Verification items for the finished model (mm, model axes). A direction names the side the tool comes from. Round coordinates to 2 decimals unless told otherwise and drop trailing zeros. Order: outer loops, then holes, each group sorted by start corner. A loop starts at its lowest first (then second) coordinate and runs counter-clockwise, first axis right, second up. Notation, with made-up numbers: M 74.5,73 L 105.5,73 A34 cw 105.5,105 Z; hole C 25,44 d7. An arc over 180 degrees is marked long. Write item = value, one per line. Start each with the question number.
from build123d import *

# Parameters (mm, degrees)
SKIZZE4_R                        = 5
SCHNITT_LINEAR_AUSTRAGEN1_DEPTH  = 32.25
SKIZZE5_R                        = 1.3
SCHNITT_LINEAR_AUSTRAGEN2_DEPTH  = 13
F_2_6_2_6_DURCHMESSER_BOHRUNG1_D = 2.6
KREISMUSTER1_COUNT               = 21


with BuildPart() as part:
    # Skizze2 → Rotation1 (revolve)
    with BuildSketch(Plane.XY, mode=Mode.PRIVATE) as rotation1_sk:
        Polygon((0, 26.075), (3.5, 26.075), (3.5, 41), (35.75, 41), (35.75, 50), (0, 50), align=None)
    rotation1 = revolve(rotation1_sk.sketch.rotate(Axis((0, 0, 0), (-1, 0, 0)), 90), axis=Axis((0, 0, 0), (-1, 0, 0)))

    # Skizze4 → Schnitt-Linear austragen1 (cut)
    with BuildSketch(Plane(origin=(35.75, 0, 0), x_dir=(0, 0, -1), z_dir=(1, 0, 0))):
        with Locations((40, 0)):
            Circle(SKIZZE4_R)
        with Locations((38.222912231, -11.790206976)):
            Circle(SKIZZE4_R)
        with Locations((33.049550973, -22.532802323)):
            Circle(SKIZZE4_R)
        with Locations((24.939592074, -31.273259299)):
            Circle(SKIZZE4_R)
        with Locations((14.613640975, -37.234949946)):
            Circle(SKIZZE4_R)
        with Locations((2.989203743, -39.888151887)):
            Circle(SKIZZE4_R)
        with Locations((-8.900837358, -38.997116487)):
            Circle(SKIZZE4_R)
        with Locations((-20, -34.641016151)):
            Circle(SKIZZE4_R)
        with Locations((-29.322074873, -27.206909511)):
            Circle(SKIZZE4_R)
        with Locations((-36.038754716, -17.355349565)):
            Circle(SKIZZE4_R)
        with Locations((-39.553233049, -5.961690647)):
            Circle(SKIZZE4_R)
        with Locations((-39.553233049, 5.961690647)):
            Circle(SKIZZE4_R)
        with Locations((-36.038754716, 17.355349565)):
            Circle(SKIZZE4_R)
        with Locations((-29.322074873, 27.206909511)):
            Circle(SKIZZE4_R)
        with Locations((-20, 34.641016151)):
            Circle(SKIZZE4_R)
        with Locations((-8.900837358, 38.997116487)):
            Circle(SKIZZE4_R)
        with Locations((2.989203743, 39.888151887)):
            Circle(SKIZZE4_R)
        with Locations((14.613640975, 37.234949946)):
            Circle(SKIZZE4_R)
        with Locations((24.939592074, 31.273259299)):
            Circle(SKIZZE4_R)
        with Locations((33.049550973, 22.532802323)):
            Circle(SKIZZE4_R)
        with Locations((38.222912231, 11.790206976)):
            Circle(SKIZZE4_R)
    schnitt_linear_austragen1 = extrude(amount=-SCHNITT_LINEAR_AUSTRAGEN1_DEPTH, mode=Mode.SUBTRACT)

    # Skizze5 → Schnitt-Linear austragen2 (cut)
    with BuildSketch(Plane(origin=(35.75, 0, 0), x_dir=(0, 0, -1), z_dir=(1, 0, 0))):
        with Locations((-46.369838758, 0)):
            Circle(SKIZZE5_R)
        with Locations((-28.91112158, 36.253399778)):
            Circle(SKIZZE5_R)
        with Locations((10.318259828, 45.207250089)):
            Circle(SKIZZE5_R)
        with Locations((41.777781131, 20.119119023)):
            Circle(SKIZZE5_R)
        with Locations((41.777781131, -20.119119023)):
            Circle(SKIZZE5_R)
        with Locations((10.318259828, -45.207250089)):
            Circle(SKIZZE5_R)
        with Locations((-28.91112158, -36.253399778)):
            Circle(SKIZZE5_R)
    schnitt_linear_austragen2 = extrude(amount=-SCHNITT_LINEAR_AUSTRAGEN2_DEPTH, mode=Mode.SUBTRACT)

    # Spiegeln1: Rotation1, Schnitt-Linear austragen1, Schnitt-Linear austragen2 across plane
    add(rotation1.mirror(Plane(origin=(0, 0, 0), x_dir=(0, 0, 1), z_dir=(1, 0, 0))))
    add(schnitt_linear_austragen1.mirror(Plane(origin=(0, 0, 0), x_dir=(0, 0, 1), z_dir=(1, 0, 0))), mode=Mode.SUBTRACT)
    add(schnitt_linear_austragen2.mirror(Plane(origin=(0, 0, 0), x_dir=(0, 0, 1), z_dir=(1, 0, 0))), mode=Mode.SUBTRACT)

    # Ø2.6 (2.6) Durchmesser Bohrung1 (through all)
    with Locations(Plane(origin=(3.5, 0, 0), x_dir=(0, 0, -1), z_dir=(1, 0, 0))):
        with Locations((40, 0)):
            f_2_6_2_6_durchmesser_bohrung1 = Hole(F_2_6_2_6_DURCHMESSER_BOHRUNG1_D / 2)

    # Kreismuster1: Ø2.6 (2.6) Durchmesser Bohrung1 ×21 about axis
    kreismuster1_axis = Axis((0, 0, 0), (1, 0, 0))
    for i in range(1, KREISMUSTER1_COUNT):
        add(f_2_6_2_6_durchmesser_bohrung1.rotate(kreismuster1_axis, i * 360 / KREISMUSTER1_COUNT), mode=Mode.SUBTRACT)


solid = part.part
1) Access from +Z, -Z, +X, -X, +Y, -Y to the whole of each face (thin tool, end or side, straight path). Record for faces 3 (the cylindrical face through (-0.05, 12.63, -37.23)), 4 (the cylindrical face through (19.85, -38.92, 22.59)), 5 (the cylindrical face through (-19.85, -44.88, -3.26)).
2) Scan lines: probe 1 along Z at (x, y) = (32.5, 1); probe 2 along X at (y, z) = (16.5, -33); probe 3 along Z at (x, y) = (9.5, 4.5). Record each from-to range of solid material in increasing order.
3) Release check for a two-part mould opening along Y. For faces 1 (the cylindrical face through (-29.34, -36.75, 27.71)), 2 (the flat face through (35.75, 18.3, -37.3)) record: pulls with the +Y half, pulls with the -Y half, needs draft (parallel to the pull), parting line crosses it, or undercut.
4) Cross-section at B-B, the plane z = 0. Enter the section's corners in (x, y) (3 decimals).
5) Cross-section at A-A, the plane x = 2. Give the number of separate pieces and of enclosed holes in the cut face, then the cut area to 3 significant figures.
6) Gauge pin test, flat ends, axial feed: P1, Ø12, axis at x = 24, z = 1, coming from the -Y side; P2, Ø12, axis at y = -39.5, z = -35, coming from the -X side; P3, Ø10, axis at x = -4, y = 7, coming from the -Z side; P4, Ø4, axis at y = 39.89, z = -2.99, coming from the +X side. Record the tip position at first contact, or that the pin passes through.
Geometry results:
q1.face_3 = +X, -X
q1.face_4 = +X
q1.face_5 = -X
q2.probe_1 = -49.99 to -44.9, 40.99 to 45.54, 47.2 to 49.99
q2.probe_2 = -3.5 to 3.5
q2.probe_3 = -49.8 to -42.18, 44.33 to 49.8
q3.face_1 = undercut
q3.face_2 = needs draft
q4.outline = M -35.75,-50 L 35.75,-50 L 35.75,-43.896 L 3.5,-43.896 L 3.5,-26.075 L -3.5,-26.075 L -3.5,-43.896 L -35.75,-43.896 Z; M -35.75,43.896 L -3.5,43.896 L -3.5,26.075 L 3.5,26.075 L 3.5,43.896 L 35.75,43.896 L 35.75,50 L -35.75,50 Z
q5.separate_pieces = 1
q5.enclosed_holes = 22
q5.area = 5,610 mm^2
q6.P1 = -50
q6.P2 = -35.75
q6.P3 = -49.96
q6.P4 = 3.5
